Could you check a few things on this model? Use its own coordinates, in mm. A direction names the side the tool comes from. Round coordinates to 2 decimals unless told otherwise and drop trailing zeros. Order: outer loops, then holes, each group sorted by start corner. A loop starts at its lowest first (then second) coordinate and runs counter-clockwise, first axis right, second up. Notation, with made-up numbers: (-27, 68.5) - (23, 68.5) arc R30 ccw to (23, 107.5) - close; hole circle Ø5 at (8, 4). An arc over 180 degrees is marked (long way). Use one line per item in the form item = value.
from build123d import *

# Parameters (mm, degrees)
F0_W     = 20
F0_H     = 20
F0_R     = 5
F0_H_2   = 40
F1_DEPTH = 100
F2_W     = 60
F2_H     = 34.6079095881
F3_DEPTH = 131.6404025087


# Not quite as in the source:
# - a feature names something its author has since deleted; it is built from what else it names


with BuildPart() as f1:
    # F0 (on Front) → F1 (new body)
    with BuildSketch(Plane.XZ):
        Polygon((-131.6394025087, 20), (-131.6394025087, 0), (-18.5843738595, 0), (137.0734572411, 0), (190.578520298, 0), (218.3605974913, 0), (218.3605974913, 20), (198.3605974913, 20), (-111.6394025087, 20), align=None)
        with Locations((-121.6394025087, 30)):
            Rectangle(F0_W, F0_H)
        with Locations((-121.6394025087, 30)):
            Circle(F0_R, mode=Mode.SUBTRACT)
        with Locations((208.3605974913, 40)):
            Rectangle(F0_W, F0_H_2)
        with Locations((208.3605974913, 51.0531589389)):
            Circle(F0_R, mode=Mode.SUBTRACT)
        Polygon((190.578520298, 0), (137.0734572411, 0), (146.9386657926, -17.7425388247), (181.5354246128, -17.7425388247), align=None)
        with Locations((163.6041871454, -9.4907971493)):
            Circle(F0_R, mode=Mode.SUBTRACT)
        Polygon((-18.5843738595, 0), (-131.6394025087, 0), (-105.3372249007, -30), (-49.1586900184, -30), align=None)
        with Locations((-77.2479574596, -19.8998747039)):
            Circle(F0_R, mode=Mode.SUBTRACT)
    extrude(amount=F1_DEPTH)

    # F2 (on Right) → F3 (cut, through all)
    with BuildSketch(Plane.YZ):
        with Locations((-50, -17.3039547941)):
            Rectangle(F2_W, F2_H)
    extrude(amount=-F3_DEPTH, mode=Mode.SUBTRACT)


solid = f1.part
Item 1: For faces 1 (the face through (31, -49, 0)), 2 (the face through (46, -49, 20)), 3 (the face through (164, -49, -17.743)), 4 (the face through (141.94, -49.3, -8.75)), which set-ups out of +Z, -Z, +X, -X, +Y, -Y let a thin tool reach every point of the face, with its end or its side?
Found:
face_1 = -Z
face_2 = +Z, +Y, -Y
face_3 = -Z, +X, +Y, -Y
face_4 = -Z, +Y, -Y
Item 2: Imagine slicing it at D-D on y = -28. Please give me the cut outline in (x, z).
Found:
outline = (-131.64, 0) - (137.07, 0) - (146.94, -17.74) - (181.54, -17.74) - (190.58, 0) - (218.36, 0) - (218.36, 60) - (198.36, 60) - (198.36, 20) - (-111.64, 20) - (-111.64, 40) - (-131.64, 40) - close; hole circle Ø10 at (-121.64, 30); hole circle Ø10 at (163.6, -9.49); hole circle Ø10 at (208.36, 51.05)
Item 3: Imagine slicing it at B-B on y = -10. Please give me the cut outline in (x, z).
Found:
outline = (-131.64, 0) - (-105.34, -30) - (-49.16, -30) - (-18.58, 0) - (137.07, 0) - (146.94, -17.74) - (181.54, -17.74) - (190.58, 0) - (218.36, 0) - (218.36, 60) - (198.36, 60) - (198.36, 20) - (-111.64, 20) - (-111.64, 40) - (-131.64, 40) - close; hole circle Ø10 at (-121.64, 30); hole circle Ø10 at (-77.25, -19.9); hole circle Ø10 at (163.6, -9.49); hole circle Ø10 at (208.36, 51.05)
Item 4: Imagine slicing it at C-C on x = 172. Please give me the cut outline in (y, z), plus the area to 3 significant figures.
Found:
outline = (-100, -17.74) - (0, -17.74) - (0, 20) - (-100, 20) - close
area = 3,770 mm2
Item 5: If we mould it in two halves opening along Y, with no side actions, what happens to faces 5 (the face through (-118.67, -89.86, -14.79)), 6 (the face through (17, 0, 2)), 7 (the face through (-74, -20, -12))? For each: released by +Y, released by -Y, zero draft, split by the parting line, or undercut.
Found:
face_5 = zero draft
face_6 = released by +Y
face_7 = undercut
Item 6: I need wall thicknesses on L1, parallel to Y at x = -38, z = -19; L2, parallel to Z at x = -104, y = -15.5; L3, parallel to Z at x = 127, y = -5. Which ranges of each line are inside material? Lowest first, please.
Found:
L1 = -100 to -80, -20 to 0
L2 = -30 to 20
L3 = 0 to 20
Item 7: Will these pins go through, and if not, where does the flat tip stop? P1, Ø9, axis at x = 163.6, z = -9.49, coming from the -Y side; P2, Ø10, axis at x = 121.5, y = -31, coming from the +Z side; P3, Ø4, axis at x = -79.5, z = 20.5, coming from the -Y side; P4, Ø3, axis at x = -15, y = -10.5, coming from the -Z side.
Found:
P1 = through
P2 = 20
P3 = -100
P4 = 0
Item 8: Imagine slicing it at A-A on z = 30. Please give me the cut outline in (x, y).
Found:
outline = (-131.64, -100) - (-126.64, -100) - (-126.64, 0) - (-131.64, 0) - close; (-116.64, -100) - (-111.64, -100) - (-111.64, 0) - (-116.64, 0) - close; (198.36, -100) - (218.36, -100) - (218.36, 0) - (198.36, 0) - close
